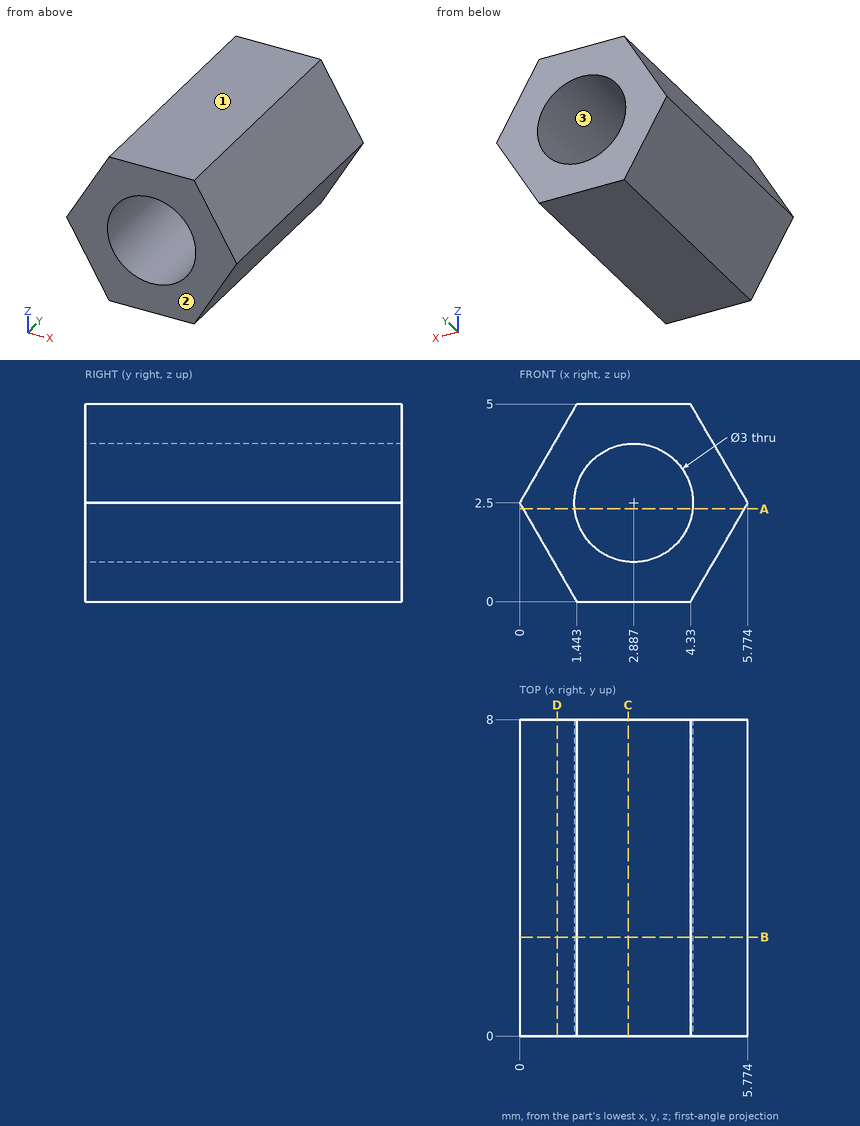
For this review, use the dimensioned drawing (mm, ordinates from the lowest corner) and the shaded views. Round coordinates to 2 decimals unless told otherwise and drop trailing zeros. Order: outer loops, then holes, each group sorted by start corner. A loop starts at its lowest first (then second) coordinate and runs counter-clockwise, first axis right, second up. Notation, with made-up numbers: M -27,78.25 L 12,78.25 A37 cw 12,114.25 Z; hole C 89.25,44.5 d11. An arc over 180 degrees is marked long. Write each question's results on one line, items separated by ' | '. Start each with the question number.
1. To check wall thickness, follow L1, parallel to Z at x = 2.85, y = 2.75; L2, parallel to Z at x = 3.45, y = 7.5; L3, parallel to X at y = 3, z = 1.3 (1 decimal). State the ranges of each line that lie inside material, in increasing order. Write a range as [from, to].
2. Draft analysis for pull direction Z (two halves, no side actions). For the marked faces 1, 2 and 3, state which applies: pulls with the +Z half, pulls with the -Z half, needs draft (parallel to the pull), parting line crosses it, or undercut.
3. Clearance check with a flat-ended pin moving along its axis: pin 1 Ø1.5 at (y, z) = (6.5, 1) entering from +X. State where the tip first meets the part, or that it passes through.
4. Add section D-D (x = 0.95). State the section outline as (y, z) points (1 decimal), then the cut area to 3 significant figures.
5. Add section C-C (x = 2.75). State the section outline as (y, z) points.
6. Add section B-B (y = 2.5). State the section outline as (x, z) points.
7. Add section A-A (z = 2.35). State the section outline as (x, y) points (1 decimal).
Output values:
1) L1: [0, 1], [4, 5] | L2: [0, 1.11], [3.89, 5] | L3: [0.7, 2], [3.8, 5.1]
2) face 1: pulls with the +Z half | face 2: needs draft | face 3: undercut
3) pin 1: x = 5.34
4) outline: M 0,0.9 L 8,0.9 L 8,4.1 L 0,4.1 Z | area: 26.3 mm^2
5) outline: M 0,0 L 8,0 L 8,1.01 L 0,1.01 Z; M 0,3.99 L 8,3.99 L 8,5 L 0,5 Z
6) outline: M 0,2.5 L 1.44,0 L 4.33,0 L 5.77,2.5 L 4.33,5 L 1.44,5 Z; hole C 2.89,2.5 d3
7) outline: M 0.1,0 L 1.4,0 L 1.4,8 L 0.1,8 Z; M 4.4,0 L 5.7,0 L 5.7,8 L 4.4,8 Z
